The model under review builds one solid part; all positions refer to its coordinate system, in mm. A direction names the side the tool comes from. Round coordinates to 2 decimals unless told otherwise and drop trailing zeros. Write each loop counter-clockwise with the first axis right and the second up, starting at its lowest first coordinate (ties: lowest second). Pieces come first, ordered by that corner, then holes. Notation, with made-up numbers: (70.5, 84) -> (84.5, 84) arc R28 ccw to (84.5, 113) -> close; hole circle Ø2 at (7.5, -27). An arc over 180 degrees is marked (long way). Answer as a JSON object with one key per item and string values. Group by question number.
1) We need section C-C, the plane z = 119. Write out the cut boundary in (x, y), then the cut area to 3 significant figures.
2) We need section A-A, the plane x = 0. Write out the cut boundary in (y, z).
3) Machinability: for faces 5 (the flat face through (-2, -8, 165)), 6 (the cylindrical face through (1.73, -7.81, -140.35)), which of the approach directions +Z, -Z, +X, -X, +Y, -Y give a long, thin tool a straight path to every point of the face, cutting with its end or side? Answer none if there is none.
4) We need section D-D, the plane z = -140.5. Write out the cut boundary in (x, y).
5) Insertion check: pin 1 Ø8 at (y, z) = (5, -27) entering from +X; pin 2 Ø10 at (x, z) = (-3, 131) entering from +Y; pin 3 Ø8 at (x, y) = (0.5, 2.5) entering from -Z; pin 4 Ø8 at (x, z) = (8, -77) entering from +Y. Each pin has a flat end and moves straight along its axis. Give the tip position at first contact, or say it passes through.
6) Mouldability with a two-part tool opening along X and no side actions: class faces 1 (the flat face through (-4, -6, -115)), 2 (the cylindrical face through (6.466, -2.681, 22.547)), 3 (the cylindrical face through (-2.38, -10.74, 2.31)), 4 (the flat face through (-2, -8, -165)) as pulls with the +X half, pulls with the -X half, needs draft (parallel to the pull), parting line crosses it, or undercut.
7) To check wall thickness, follow probe 1 along Y at (x, z) = (0, -149.5); probe 2 along Y at (x, z) = (0, 58.5); probe 3 along X at (y, z) = (1, -125.5). State the ranges of each line that lie inside material, in increasing order. Write a range as [from, to].
from build123d import *

# Parameters (mm, degrees)
SZKIC1_R                    = 11
SZKIC1_R_2                  = 7
DODANIE_WYCI_GNI_CIE1_DEPTH = 165
SZKIC2_R                    = 8
WYTNIJ_WYCI_GNI_CIE1_DEPTH  = 50
SFAZOWANIE1_SIZE            = 1


with BuildPart() as part:
    # Szkic1 → Dodanie-wyciągnięcie1 (new, symmetric)
    with BuildSketch(Plane.XY):
        Circle(SZKIC1_R)
        Circle(SZKIC1_R_2, mode=Mode.SUBTRACT)
    extrude(amount=DODANIE_WYCI_GNI_CIE1_DEPTH, both=True)

    # Szkic2 → Wytnij-wyciągnięcie1 (cut)
    with BuildSketch(Plane(origin=(0, 0, -165), x_dir=(-1, 0, 0), z_dir=(0, 0, -1))):
        Circle(SZKIC2_R)
    extrude(amount=-WYTNIJ_WYCI_GNI_CIE1_DEPTH, mode=Mode.SUBTRACT)

    # Sfazowanie1
    sfazowanie1_edges = [part.edges().sort_by_distance(p)[0] for p in [
        (-7, 0, 165),
    ]]
    chamfer(sfazowanie1_edges, length=SFAZOWANIE1_SIZE)


solid = part.part
Here are the results:
{
 "1": {"outline": "circle Ø22 at (0, 0); hole circle Ø14 at (0, 0)", "area": "226 mm^2"},
 "2": {"outline": "(-11, -165) -> (-8, -165) -> (-8, -115) -> (-7, -115) -> (-7, 164) -> (-8, 165) -> (-11, 165) -> close; (7, -115) -> (8, -115) -> (8, -165) -> (11, -165) -> (11, 165) -> (8, 165) -> (7, 164) -> close"},
 "3": {"face 5": "+Z, +X, -X, +Y, -Y", "face 6": "-Z"},
 "4": {"outline": "circle Ø22 at (0, 0); hole circle Ø16 at (0, 0)"},
 "5": {"pin 1": "stops at x = 10.95", "pin 2": "stops at y = 11", "pin 3": "passes through", "pin 4": "stops at y = 10.25"},
 "6": {"face 1": "undercut", "face 2": "undercut", "face 3": "parting line crosses it", "face 4": "needs draft"},
 "7": {"probe 1": "y = [-11, -8], [8, 11]", "probe 2": "y = [-11, -7], [7, 11]", "probe 3": "x = [-10.95, -7.94], [7.94, 10.95]"}
}
